Verification items for the finished model (mm, model axes). Face numbers are marked on the shaded views. A direction names the side the tool comes from. Coordinates: 2 decimals unless noted, no trailing zeros. Loops run counter-clockwise (first coordinate to the right, second up) from the corner with the lowest first, then second, coordinate; pieces in that order, holes last. Notation, with made-up numbers: (81.5, 35.25) - (117.5, 35.25) arc R22 cw to (117.5, 49.25) - close; hole circle Ø8 at (-22, 76.5). An arc over 180 degrees is marked (long way). Answer as CSV lines item,"result". Start each with the question number.
1. Cross-section at A-A (z = 6). Enter the section's corners in (x, y).
2. Cross-section at C-C (y = -7). Enter the section's corners in (x, z), plus the area to 3 significant figures.
3. Release check for a two-part mould opening along Z. For the marked faces 3, 4, 5 and 6 record: pulls with the +Z half, pulls with the -Z half, needs draft (parallel to the pull), parting line crosses it, or undercut.
4. Material ranges on line 1 (Z direction, x = -9.3, y = 11.9); line 2 (Y direction, x = -10.5, z = 8.25); line 3 (Z direction, x = 2, y = 4.25), recorded low to high. Write a range as [from, to].
5. Gauge pin test, flat ends, axial feed: P1, Ø1.6, axis at x = 0, z = 0.5, coming from the +Y side; P2, Ø1.6, axis at y = -9, z = 0.5, coming from the -X side; P3, Ø4, axis at x = 8.5, y = 4, coming from the +Z side. Record the tip position at first contact, or that the pin passes through.
6. Set-up check for the marked faces 1 and 2: record each of +Z, -Z, +X, -X, +Y, -Y from which the full face is reachable in a straight line by a thin tool's end or side.
```python
from build123d import *

# Parameters (mm, degrees)
PAD_DEPTH    = 1.5
SKETCH001_W  = 26.017304
SKETCH001_H  = 2.649366
PAD001_DEPTH = 8
SKETCH002_R  = 1.6
POCKET_DEPTH = 2.650366


with BuildPart() as part:
    # Sketch → Pad (new body)
    with BuildSketch(Plane.XY):
        with BuildLine():
            Line((-13, 12.5), (13, 12.5))
            Line((13, 12.5), (13, -12.5))
            Line((13, -12.5), (9.6, -12.5))
            Line((9.6, -7.500992), (9.6, -12.5))
            ThreePointArc((9.6, -7.500992), (7.5, -5.4), (5.4, -7.500992))
            Line((5.4, -7.500992), (5.4, -12.5))
            Line((5.4, -12.5), (-5.40282, -12.5))
            Line((-5.40282, -7.608787), (-5.40282, -12.5))
            ThreePointArc((-5.40282, -7.608787), (-7.5, -5.4), (-9.59718, -7.608787))
            Line((-9.59718, -7.608787), (-9.59718, -12.5))
            Line((-9.59718, -12.5), (-13, -12.5))
            Line((-13, -12.5), (-13, 12.5))
        make_face()
    extrude(amount=PAD_DEPTH)

    # Sketch001 → Pad001 (new body)
    with BuildSketch(Plane.XY.offset(1.5)):
        with Locations((-0.008652, 11.17938)):
            Rectangle(SKETCH001_W, SKETCH001_H)
    extrude(amount=PAD001_DEPTH)

    # Sketch002 → Pocket (cut, through all)
    with BuildSketch(Plane.XZ.offset(-9.854697)):
        with Locations((-9.3, 6)):
            Circle(SKETCH002_R)
        with Locations((9.3, 6)):
            Circle(SKETCH002_R)
    extrude(amount=-POCKET_DEPTH, mode=Mode.SUBTRACT)


solid = part.part
```
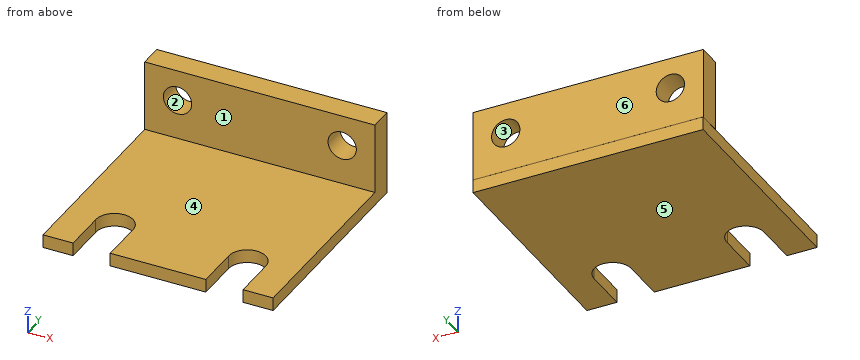
Values follow:
1,outline,"(-13.02, 9.85) - (-10.9, 9.85) - (-10.9, 12.5) - (-13.02, 12.5) - close; (-7.7, 9.85) - (7.7, 9.85) - (7.7, 12.5) - (-7.7, 12.5) - close; (10.9, 9.85) - (13, 9.85) - (13, 12.5) - (10.9, 12.5) - close"
2,outline,"(-13, 0) - (-9.54, 0) - (-9.54, 1.5) - (-13, 1.5) - close; (-5.46, 0) - (5.46, 0) - (5.46, 1.5) - (-5.46, 1.5) - close; (9.54, 0) - (13, 0) - (13, 1.5) - (9.54, 1.5) - close"
2,area,"26.8 mm²"
3,face 3,"undercut"
3,face 4,"pulls with the +Z half"
3,face 5,"pulls with the -Z half"
3,face 6,"needs draft"
4,line 1,"z = [0, 4.4], [7.6, 9.5]"
4,line 2,"y = [9.85, 12.5]"
4,line 3,"z = [0, 1.5]"
5,P1,"stops at y = 12.5"
5,P2,"stops at x = -13"
5,P3,"stops at z = 1.5"
6,face 1,"+Z, +X, -X, -Y"
6,face 2,"+Y, -Y"
